from build123d import *

# Parameters (mm, degrees)
SKETCH2_R           = 15.875
BOSS_EXTRUDE1_DEPTH = 29.972
SKETCH3_R           = 12.065
CUT_EXTRUDE1_DEPTH  = 24.13
CUT_EXTRUDE2_REACH  = 39.448
SKETCH4_R           = 2.54


with BuildPart() as part:
    # Sketch2 → Boss-Extrude1 (new body)
    with BuildSketch(Plane(origin=(0, 0, 0), x_dir=(1, 0, 0), z_dir=(0, 1, 0))):
        with Locations(Location((0, 0, 0), (0, 0, 270))):
            Circle(SKETCH2_R)
    extrude(amount=BOSS_EXTRUDE1_DEPTH)

    # Sketch3 → Cut-Extrude1 (cut)
    with BuildSketch(Plane.XZ):
        with Locations(Location((0, 0, 0), (0, 0, 270))):
            Circle(SKETCH3_R)
    extrude(amount=-CUT_EXTRUDE1_DEPTH, mode=Mode.SUBTRACT)

    # Sketch4 → Cut-Extrude2 (cut, up to next)
    with BuildSketch(Plane(origin=(0, 29.972, 0), x_dir=(1, 0, 0), z_dir=(0, 1, 0)), mode=Mode.PRIVATE) as cut_extrude2_sk1:
        with Locations(Location((0, 0, 0), (0, 0, 270))):
            Circle(SKETCH4_R)
    cut_extrude2_tool1 = extrude(cut_extrude2_sk1.sketch, amount=-CUT_EXTRUDE2_REACH, mode=Mode.PRIVATE) & part.part
    add(cut_extrude2_tool1.solids().sort_by_distance((0, 29.972, 0))[0], mode=Mode.SUBTRACT)


solid = part.part
The model under review builds one solid part; all positions refer to its coordinate system, in mm. A direction names the side the tool comes from. Round coordinates to 2 decimals unless told otherwise and drop trailing zeros. Loops run counter-clockwise (first coordinate to the right, second up) from the corner with the lowest first, then second, coordinate; pieces in that order, holes last. Notation, with made-up numbers: M 88,46 L 93,46 A22 cw 93,75 Z; hole C 59.25,72.25 d6. An arc over 180 degrees is marked long. Answer as CSV lines item,"result". Start each with the question number.
Item 1: For faces 1 (the face through (3, 24.13, 0)), 2 (the face through (2.52, 27.09, -0.33)), list the 3-axis set-ups (+Z, -Z, +X, -X, +Y, -Y) from which the entire face can be reached by the end or side of a thin tool; tool diameter is ignored.
Item 2: Consider section A-A (x = 0). Write out the cut boundary in (y, z) (3 decimals), then the cut area to 3 significant figures.
Item 3: Consider section C-C (y = 23.25). Write out the cut boundary in (x, z) (3 decimals), then the cut area to 3 significant figures.
Item 4: Consider section B-B (z = 0). Write out the cut boundary in (x, y) (3 decimals), then the cut area to 3 significant figures.
Item 5: Insertion check: P1, Ø1.5, axis at x = -8.5, y = 21, coming from the +Z side; P2, Ø8, axis at y = 10.5, z = -1.5, coming from the -X side (3 decimals); P3, Ø7, axis at x = -1.5, z = 2, coming from the -Y side; P4, Ø1, axis at y = 5.5, z = 4, coming from the -X side. Each pin has a flat end and moves straight along its axis. Give the tip position at first contact, or say it passes through.
Item 6: Mouldability with a two-part tool opening along Z and no side actions: class faces 3 (the face through (3.62, 11.9, -11.51)), 4 (the face through (-15.497, 14.776, -3.441)), 5 (the face through (6, 0, 11)) as released by +Z, released by -Z, zero draft, split by the parting line, or undercut.
Item 7: Wall thickness on line 1 (X direction, y = 13.5, z = 0) (3 decimals); line 2 (X direction, y = 25.55, z = 0) (3 decimals); line 3 (Y direction, x = -8, z = 4): over which ranges is each line inside the solid? List them lowest first. Write a range as [from, to].
Item 8: Consider section D-D (z = 10.5). Write out the cut boundary in (x, y), then the cut area to 3 significant figures.
Answer:
1,face 1,"-Y"
1,face 2,"+Y, -Y"
2,outline,"M 0,-15.875 L 29.972,-15.875 L 29.972,-2.54 L 24.13,-2.54 L 24.13,-12.065 L 0,-12.065 Z; M 0,12.065 L 24.13,12.065 L 24.13,2.54 L 29.972,2.54 L 29.972,15.875 L 0,15.875 Z"
2,area,"340 mm^2"
3,outline,"C 0,0 d31.75; hole C 0,0 d24.13"
3,area,"334 mm^2"
4,outline,"M -15.875,0 L -12.065,0 L -12.065,24.13 L -2.54,24.13 L -2.54,29.972 L -15.875,29.972 Z; M 2.54,24.13 L 12.065,24.13 L 12.065,0 L 15.875,0 L 15.875,29.972 L 2.54,29.972 Z"
4,area,"340 mm^2"
5,P1,"stops at z = 13.85"
5,P2,"stops at x = -15.875"
5,P3,"stops at y = 24.13"
5,P4,"stops at x = -15.48"
6,face 3,"undercut"
6,face 4,"split by the parting line"
6,face 5,"zero draft"
7,line 1,"x = [-15.875, -12.065], [12.065, 15.875]"
7,line 2,"x = [-15.875, -2.54], [2.54, 15.875]"
7,line 3,"y = [24.13, 29.97]"
8,outline,"M -11.91,0 L -5.94,0 L -5.94,24.13 L 5.94,24.13 L 5.94,0 L 11.91,0 L 11.91,29.97 L -11.91,29.97 Z"
8,area,"427 mm^2"
